Work out the finished part from the listing and answer in its coordinate system (mm). A direction names the side the tool comes from. Give positions to 0.01 mm unless a question says otherwise; leave off trailing zeros. Order: outer loops, then holes, each group sorted by start corner. A loop starts at its lowest first (then second) coordinate and runs counter-clockwise, first axis right, second up. Notation, with made-up numbers: M 31,88 L 51,88 A22 cw 51,116 Z; hole C 89.5,-3 d9. An arc over 180 degrees is marked long. One line per item, written item: value.
from build123d import *

# Parameters (mm, degrees)
F1_DEPTH = 10.16
F3_D     = 2.286
F4_W     = 19.431
F4_H     = 5.969
F4_R     = 1.3254329065
F4_W_2   = 6.35
F4_H_2   = 2.794
F4_R_2   = 1.3633247541
F5_DEPTH = 1.016
F6_R     = 0.381


with BuildPart() as f1:
    # F0 (on Front) → F1 (new body)
    with BuildSketch(Plane.XZ):
        Polygon((-7.366, 1.016), (-7.366, 0), (0, 0), (0, 5.969), (19.431, 5.969), (19.431, 0), (26.797, 0), (26.797, 1.016), (20.447, 1.016), (20.447, 6.985), (-1.016, 6.985), (-1.016, 1.016), align=None)
    extrude(amount=F1_DEPTH)

    # F3 (through all)
    with Locations(Plane.XY.offset(1.016)):
        with Locations((-4.191, -5.08), (23.622, -5.08)):
            Hole(F3_D / 2)

    # F4 (on face) → F5 (join)
    with BuildSketch(Plane.XZ.offset(10.16)):
        with Locations((9.7155, 2.9845)):
            Rectangle(F4_W, F4_H)
        with Locations((2.5069266703, 3.048)):
            Circle(F4_R, mode=Mode.SUBTRACT)
        with Locations((9.8729266703, 3.048)):
            Rectangle(F4_W_2, F4_H_2, mode=Mode.SUBTRACT)
        with Locations((17.2389266703, 3.0497561675)):
            Circle(F4_R_2, mode=Mode.SUBTRACT)
    extrude(amount=-F5_DEPTH)

    # F6
    f6_edges = [f1.edges().sort_by_distance(p)[0] for p in [
        (20.447, -5.08, 6.985),
        (-1.016, -5.08, 6.985),
        (9.7155, 0, 6.985),
        (9.7155, -10.16, 6.985),
        (-1.016, -10.16, 4.0005),
        (-1.016, -5.08, 1.016),
        (-4.191, -10.16, 1.016),
        (-7.366, -10.16, 0.508),
        (-7.366, -5.08, 1.016),
        (-7.366, 0, 0.508),
        (-4.191, 0, 1.016),
        (0, 0, 2.9845),
        (9.7155, 0, 5.969),
        (19.431, 0, 2.9845),
        (20.447, 0, 4.0005),
        (20.447, -5.08, 1.016),
        (23.622, 0, 1.016),
        (26.797, 0, 0.508),
        (26.797, -5.08, 1.016),
        (26.797, -10.16, 0.508),
        (23.622, -10.16, 1.016),
        (20.447, -10.16, 4.0005),
        (-1.016, 0, 4.0005),
    ]]
    fillet(f6_edges, radius=F6_R)


solid = f1.part
(1) Determine the mould class of faces 4 (the cylindrical face through (22.53, -4.74, 0.5)), 5 (the flat face through (10, -10, 1.651)), 6 (the cylindrical face through (-5.247, -5.518, 0.501)), 7 (the flat face through (9, -10.16, 5)) for opening direction Y: pulls with the +Y half, pulls with the -Y half, needs draft (parallel to the pull), parting line crosses it, or undercut.
Findings:
face 4: undercut
face 5: needs draft
face 6: undercut
face 7: pulls with the -Y half
(2) Section B-B, the plane x = 11 is taken. Give the vertices of the cut face in (y, z) (3 decimals), then the cut area to 3 significant figures.
Findings:
outline: M -10.16,0 L -9.144,0 L -9.144,1.651 L -10.16,1.651 Z; M -10.16,4.445 L -9.144,4.445 L -9.144,5.969 L -0.381,5.969 A0.381 ccw 0,6.35 L 0,6.604 A0.381 ccw -0.381,6.985 L -9.779,6.985 A0.381 ccw -10.16,6.604 Z
area: 13.5 mm^2
(3) Section C-C, the plane z = 3.5 is taken. Give the vertices of the cut face in (x, y) (3 decimals).
Findings:
outline: M -1.016,-9.779 A0.381 ccw -0.635,-10.16 L 1.261,-10.16 L 1.261,-9.144 L 0,-9.144 L 0,-0.381 A0.381 ccw -0.381,0 L -0.635,0 A0.381 ccw -1.016,-0.381 Z; M 3.753,-10.16 L 6.698,-10.16 L 6.698,-9.144 L 3.753,-9.144 Z; M 13.048,-10.16 L 15.952,-10.16 L 15.952,-9.144 L 13.048,-9.144 Z; M 18.526,-10.16 L 20.066,-10.16 A0.381 ccw 20.447,-9.779 L 20.447,-0.381 A0.381 ccw 20.066,0 L 19.812,0 A0.381 ccw 19.431,-0.381 L 19.431,-9.144 L 18.526,-9.144 Z
(4) Which of the six approach directions +Z, -Z, +X, -X, +Y, -Y give full straight-line access (tool end or side, diameter ignored) to faces 1 (the flat face through (-5, -4, 1.016)), 2 (the flat face through (10, -9.144, 1)), 3 (the flat face through (20.447, -5, 4))?
Findings:
face 1: +Z, -X, +Y, -Y
face 2: -Z, +Y
face 3: +Z, +X, +Y, -Y
(5) Given P1, Ø1.1, axis at y = -9.5, z = 3.5, coming from the -X side; P2, Ø4.5, axis at x = 24, y = -6, coming from the +Z side; P3, Ø1.6, axis at y = -5, z = 5, coming from the +X side; P4, Ø1.8, axis at x = -4.191, y = -5.08, coming from the +Z side, each flat-ended and moving along its own axis, determine where each tip first touches the part or whether it passes through.
Findings:
P1: stops at x = -1.02
P2: stops at z = 1.02
P3: stops at x = 20.45
P4: passes through
(6) Section A-A, the plane y = -5.08 is taken. Give the vertices of the cut face in (x, z) (3 decimals).
Findings:
outline: M -7.366,0 L -5.334,0 L -5.334,1.016 L -6.985,1.016 A0.381 ccw -7.366,0.635 Z; M -3.048,0 L 0,0 L 0,5.969 L 19.431,5.969 L 19.431,0 L 22.479,0 L 22.479,1.016 L 20.828,1.016 A0.381 cw 20.447,1.397 L 20.447,6.604 A0.381 ccw 20.066,6.985 L -0.635,6.985 A0.381 ccw -1.016,6.604 L -1.016,1.397 A0.381 cw -1.397,1.016 L -3.048,1.016 Z; M 24.765,0 L 26.797,0 L 26.797,0.635 A0.381 ccw 26.416,1.016 L 24.765,1.016 Z
(7) Find the intervals of material crossed by probe 1 along X at (y, z) = (-5.25, 2.75); probe 2 along Z at (x, y) = (12.5, -3.75) (3 decimals); probe 3 along Z at (x, y) = (-1.5, -7), in increasing order. Write a range as from..to.
Findings:
probe 1: x = -1.02..0, 19.43..20.45
probe 2: z = 5.969..6.985
probe 3: z = 0..1.02
(8) Section D-D, the plane y = -8 is taken. Give the vertices of the cut face in (x, z) (3 decimals), then the cut area to 3 significant figures.
Findings:
outline: M -7.366,0 L 0,0 L 0,5.969 L 19.431,5.969 L 19.431,0 L 26.797,0 L 26.797,0.635 A0.381 ccw 26.416,1.016 L 20.828,1.016 A0.381 cw 20.447,1.397 L 20.447,6.604 A0.381 ccw 20.066,6.985 L -0.635,6.985 A0.381 ccw -1.016,6.604 L -1.016,1.397 A0.381 cw -1.397,1.016 L -6.985,1.016 A0.381 ccw -7.366,0.635 Z
area: 46.8 mm^2
